Source: CAD feature listing. Evaluate the final solid. Frame: model axes, mm. A direction names the side the tool comes from. Give positions to 0.01 mm unless a question says otherwise; leave off trailing zeros. Write each loop counter-clockwise with the first axis right and the second up, starting at its lowest first coordinate (ties: lowest second). Pieces come first, ordered by that corner, then holes.
```python
from build123d import *

# Parameters (mm, degrees)
SKETCH_1_W      = 50
SKETCH_1_H      = 15
SKETCH_1_R      = 2.25
EXTRUDE_1_DEPTH = 3
SKETCH_4_W      = 6
SKETCH_4_H      = 6
SKETCH_4_R      = 2
CHAMFER_1_SIZE  = 0.5


with BuildPart() as part:
    # Эскиз1 → Бобышка-Вытянуть1 (new body)
    with BuildSketch(Plane.XY):
        Rectangle(SKETCH_1_W, SKETCH_1_H)
        with Locations((17.25, 0)):
            Circle(SKETCH_1_R, mode=Mode.SUBTRACT)
        with Locations((-17.25, 0)):
            Circle(SKETCH_1_R, mode=Mode.SUBTRACT)
    extrude(amount=EXTRUDE_1_DEPTH)

    # По траектории1: sweep along a path in Эскиз5
    with BuildLine(Plane.ZY) as sweep_1_path:
        Line((6, 7.5), (6, 2.5))
        ThreePointArc((6, 2.5), (8.928932188, -4.571067812), (16, -7.5))
        Line((16, -7.5), (41, -7.5))
    # Эскиз4 → По траектории1 (sweep)
    with BuildSketch(Plane(origin=(0, 7.5, 0), x_dir=(1, 0, 0), z_dir=(0, 1, 0))):
        with Locations((0, -6)):
            Rectangle(SKETCH_4_W, SKETCH_4_H)
        with Locations((0, -6)):
            Circle(SKETCH_4_R, mode=Mode.SUBTRACT)
    sweep(path=sweep_1_path.line)

    # Фаска1
    chamfer_1_edges = [part.edges().sort_by_distance(p)[0] for p in [
        (3, -7.5, 41),
        (0, -10.5, 41),
        (-3, -7.5, 41),
        (0, -4.5, 41),
    ]]
    chamfer(chamfer_1_edges, length=CHAMFER_1_SIZE)


solid = part.part
```
1. Pull-direction query (Y, two-part tool) for faces 1 (the flat face through (0, 7.5, 2)), 2 (the cylindrical face through (19.396, 0.676, 1.479)), 3 (the cylindrical face through (-0.26, -5.517, 28.675)), 4 (the flat face through (-25, 0, 1)); classes: pulls with the +Y half, pulls with the -Y half, needs draft (parallel to the pull), parting line crosses it, or undercut.
2. Section query D-D (y = 1.25). Give the number of separate pieces and of enclosed holes in the cut face, plus the area to 3 significant figures.
3. Section query B-B (y = 4.5). Return loops of the section in (x, z).
4. Pin query (flat end, axial travel): P1, Ø1.8, axis at x = 0, z = 22.5, coming from the +Y side; P2, Ø3, axis at x = 2.5, y = 4.5, coming from the +Z side; P3, Ø1.5, axis at x = -8, z = 1.5, coming from the -Y side. Return the tip coordinate at first contact, or that it passes through.
5. Access query for faces 5 (the cylindrical face through (0, 5, 8)), 6 (the flat face through (0, 5, 9)), 7 (the flat face through (3, -6, 22)), 8 (the flat face through (25, 0, 1)), 9 (the flat face through (-3, -6, 17)). Directions: +Z, -Z, +X, -X, +Y, -Y. A direction counts if a zero-diameter tool reaches every point of the face in a straight line with its end or side. Return the directions, or none.
6. Section query A-A (x = 0). Return loops of the section in (y, z), plus the area to 3 significant figures.
7. Section query C-C (z = 35). Return loops of the section in (x, y), plus the area to 3 significant figures.
8. Line query: probe 1 along Z at (x, y) = (-1, -2.75); probe 2 along Z at (x, y) = (0, 3.7); probe 3 along Y at (x, z) = (-17.25, 2.4). Output: solid intervals per line, ascending.
The answers:
1. face 1: pulls with the +Y half
1. face 2: undercut
1. face 3: undercut
1. face 4: needs draft
2. separate pieces: 4
2. enclosed holes: 1
2. area: 151 mm2
3. outline: (-25, 0) - (25, 0) - (25, 3) - (3, 3) - (3, 9) - (-3, 9) - (-3, 3) - (-25, 3) - close; hole circle Ø4 at (0, 6)
4. P1: stops at y = -4.5
4. P2: stops at z = 9
4. P3: stops at y = -7.5
5. face 5: +Y
5. face 6: +Z, +X, -X, +Y
5. face 7: +Z, +X, +Y, -Y
5. face 8: +Z, -Z, +X, +Y, -Y
5. face 9: +Z, -X, +Y, -Y
6. outline: (-10.5, 16) arc R13 ccw to (2.5, 3) - (-7.5, 3) - (-7.5, 0) - (7.5, 0) - (7.5, 4) - (2.5, 4) arc R12 cw to (-9.5, 16) - (-9.5, 41) - (-10, 41) - (-10.5, 40.5) - close; (-5.5, 16) arc R8 ccw to (2.5, 8) - (7.5, 8) - (7.5, 9) - (2.5, 9) arc R7 cw to (-4.5, 16) - (-4.5, 40.5) - (-5, 41) - (-5.5, 41) - close
6. area: 136 mm2
7. outline: (-3, -10.5) - (3, -10.5) - (3, -4.5) - (-3, -4.5) - close; hole circle Ø4 at (0, -7.5)
7. area: 23.4 mm2
8. probe 1: z = 0 to 3, 4.11 to 5.51, 9.61 to 11.37
8. probe 2: z = 0 to 4, 8 to 9
8. probe 3: y = -7.5 to -2.25, 2.25 to 7.5
